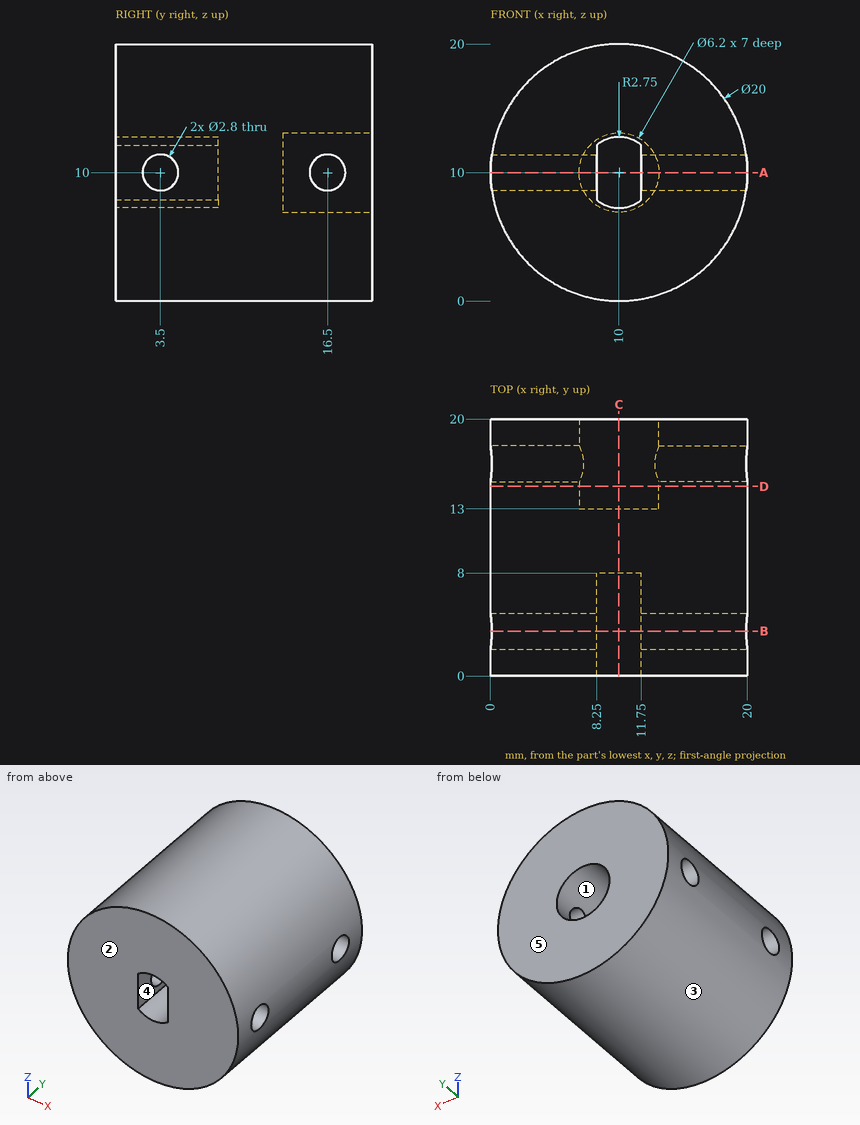
Print and shaded views of the part. All mm, measured from the part's lowest x, y and z. A direction names the side the tool comes from. Round coordinates to 2 decimals unless told otherwise and drop trailing zeros. Write each loop counter-clockwise with the first axis right and the second up, starting at its lowest first coordinate (ties: lowest second). Pieces come first, ordered by that corner, then holes. Notation, with made-up numbers: (5, 58.5) -> (54, 58.5) arc R24 cw to (54, 87.5) -> close; hole circle Ø1 at (-31.5, 46.25). An arc over 180 degrees is marked (long way). Answer in a Markdown table with one row per item. Add a question column.
Item 1: Mould opens along Z. For the marked faces 1, 2 and 3 say: pulls with the +Z half, pulls with the -Z half, needs draft (parallel to the pull), parting line crosses it, or undercut.
Item 2: Drop flat-ended pins along their axis: pin 1 Ø10 at (y, z) = (2.5, 2.5) entering from -X; pin 2 Ø1.9 at (x, z) = (11, 11.5) entering from +Y; pin 3 Ø1.7 at (y, z) = (16.5, 10) entering from +X; pin 4 Ø1 at (y, z) = (3, 3.5) entering from +X. Give the stop position or say it passes through.
Item 3: Drill centre lines: line 1 (Y direction, x = 17.5, z = 9.5); line 2 (Y direction, x = 17.5, z = 9.75); line 3 (Z direction, x = 10, y = 15). Where is each one in solid material? Low to high. Write a range as from..to.
Item 4: Saw through at D-D, the plane y = 14.75. Write the cut outline in (x, z).
Item 5: Which spindle directions (+Z, -Z, +X, -X, +Y, -Y) get a long thin tool onto all of the face, cutting with end or side? Do the marked faces 4 and 5. Say none if no direction does.
Item 6: Saw through at B-B, the plane y = 3.5. Write the cut outline in (x, z), then the cut area to 3 significant figures.
Item 7: Saw through at C-C, the plane x = 10. Write the cut outline in (y, z), then the cut area to 3 significant figures.
Item 8: Saw through at A-A, the plane z = 10. Write the cut outline in (x, y).
Findings below:
| question | item | result |
|---|---|---|
| 1 | face 1 | undercut |
| 1 | face 2 | needs draft |
| 1 | face 3 | parting line crosses it |
| 2 | pin 1 | stops at x = 0.32 |
| 2 | pin 2 | stops at y = 13 |
| 2 | pin 3 | passes through |
| 2 | pin 4 | stops at x = 18 |
| 3 | line 1 | y = 0..2.19, 4.81..15.19, 17.81..20 |
| 3 | line 2 | y = 0..2.12, 4.88..15.12, 17.88..20 |
| 3 | line 3 | z = 0..6.9, 13.1..20 |
| 4 | outline | circle Ø20 at (10, 10); hole circle Ø6.2 at (10, 10) |
| 5 | face 4 | -Y |
| 5 | face 5 | +Z, -Z, +X, -X, +Y |
| 6 | outline | (0.1, 8.6) arc R10 ccw to (19.9, 8.6) -> (11.75, 8.6) -> (11.75, 7.88) arc R2.75 cw to (8.25, 7.88) -> (8.25, 8.6) -> close; (0.1, 11.4) -> (8.25, 11.4) -> (8.25, 12.12) arc R2.75 cw to (11.75, 12.12) -> (11.75, 11.4) -> (19.9, 11.4) arc R10 ccw to start |
| 6 | area | 250 mm^2 |
| 7 | outline | (0, 0) -> (20, 0) -> (20, 6.9) -> (13, 6.9) -> (13, 13.1) -> (20, 13.1) -> (20, 20) -> (0, 20) -> (0, 12.75) -> (8, 12.75) -> (8, 7.25) -> (0, 7.25) -> close |
| 7 | area | 313 mm^2 |
| 8 | outline | (0, 0) -> (8.25, 0) -> (8.25, 2.1) -> (0, 2.1) -> close; (0, 4.9) -> (8.25, 4.9) -> (8.25, 8) -> (11.75, 8) -> (11.75, 4.9) -> (20, 4.9) -> (20, 15.1) -> (13.1, 15.1) -> (13.1, 13) -> (6.9, 13) -> (6.9, 15.1) -> (0, 15.1) -> close; (0, 17.9) -> (6.9, 17.9) -> (6.9, 20) -> (0, 20) -> close; (11.75, 0) -> (20, 0) -> (20, 2.1) -> (11.75, 2.1) -> close; (13.1, 17.9) -> (20, 17.9) -> (20, 20) -> (13.1, 20) -> close |
